Geometry check sheet. Reference: the model listing, model coordinates, mm. A direction names the side the tool comes from. Round coordinates to 2 decimals unless told otherwise and drop trailing zeros. Order: outer loops, then holes, each group sorted by start corner. A loop starts at its lowest first (then second) coordinate and runs counter-clockwise, first axis right, second up. Notation, with made-up numbers: (74, -26.5) - (120, -26.5) arc R33 ccw to (120, 1.5) - close; hole circle Ø3 at (-34.75, -28.5). An arc over 180 degrees is marked (long way). Answer as CSV lines item,"result". Start each with the question number.
```python
from build123d import *

# Parameters (mm, degrees)
SKETCH1_W           = 32
SKETCH1_H           = 22
BOSS_EXTRUDE1_DEPTH = 20
SKETCH2_R           = 4.65
BOSS_EXTRUDE2_DEPTH = 15
SKETCH3_W           = 30
SKETCH3_H           = 20
CUT_EXTRUDE1_DEPTH  = 19
SKETCH4_R           = 2.5
CUT_EXTRUDE2_DEPTH  = 28.166155414
FILLET1_R           = 1
FILLET2_R           = 1
SKETCH5_W           = 30
SKETCH5_H           = 20
SKETCH5_W_2         = 28
SKETCH5_H_2         = 18
BOSS_EXTRUDE3_DEPTH = 14
CUT_EXTRUDE3_REACH  = 50.683
SKETCH8_W           = 8
SKETCH8_H           = 5


with BuildPart() as part:
    # Sketch1 → Boss-Extrude1 (new body)
    with BuildSketch(Plane(origin=(0, 0, 0), x_dir=(1, 0, 0), z_dir=(0, 1, 0))):
        Rectangle(SKETCH1_W, SKETCH1_H)
    extrude(amount=BOSS_EXTRUDE1_DEPTH)

    # Sketch2 → Boss-Extrude2 (add)
    with BuildSketch(Plane(origin=(0, 20, 0), x_dir=(1, 0, 0), z_dir=(0, 1, 0))):
        with Locations(Location((0, 0, 0), (0, 0, 270))):
            Circle(SKETCH2_R)
    extrude(amount=BOSS_EXTRUDE2_DEPTH)

    # Sketch3 → Cut-Extrude1 (cut)
    with BuildSketch(Plane.XZ):
        Rectangle(SKETCH3_W, SKETCH3_H)
    extrude(amount=-CUT_EXTRUDE1_DEPTH, mode=Mode.SUBTRACT)

    # Sketch4 → Cut-Extrude2 (cut, through all)
    with BuildSketch(Plane.XZ.offset(-19)):
        with Locations(Location((0, 0, 0), (0, 0, 270))):
            Circle(SKETCH4_R)
    extrude(amount=-CUT_EXTRUDE2_DEPTH, mode=Mode.SUBTRACT)

    # Fillet1
    fillet1_edges = [part.edges().sort_by_distance(p)[0] for p in [
        (0, 35, -4.65),
    ]]
    fillet(fillet1_edges, radius=FILLET1_R)

    # Fillet2
    fillet2_edges = [part.edges().sort_by_distance(p)[0] for p in [
        (0, 19, 2.5),
    ]]
    fillet(fillet2_edges, radius=FILLET2_R)

    # Sketch5 → Boss-Extrude3 (add)
    with BuildSketch(Plane.XZ.offset(-19)):
        Rectangle(SKETCH5_W, SKETCH5_H)
        Rectangle(SKETCH5_W_2, SKETCH5_H_2, mode=Mode.SUBTRACT)
    extrude(amount=BOSS_EXTRUDE3_DEPTH)

    # Cut-Extrude3: up to this face of the body (flat: up to its plane)
    cut_extrude3_end = Plane(part.part.faces().sort_by_distance((14, 12, 0))[0])
    # Sketch8 → Cut-Extrude3 (cut, up to the picked face)
    with BuildSketch(Plane(origin=(16, 0, 0), x_dir=(0, 0, -1), z_dir=(1, 0, 0)), mode=Mode.PRIVATE) as cut_extrude3_sk1:
        with Locations((0, 5)):
            Rectangle(SKETCH8_W, SKETCH8_H)
    cut_extrude3_tool1 = split(extrude(cut_extrude3_sk1.sketch, amount=-CUT_EXTRUDE3_REACH, mode=Mode.PRIVATE), bisect_by=cut_extrude3_end, keep=Keep.BOTH, mode=Mode.PRIVATE)
    add(cut_extrude3_tool1.solids().sort_by(Axis((16, 5, 0), (-1, 0, 0)))[0], mode=Mode.SUBTRACT)


solid = part.part
```
1. Section check B-B on z = 0. Record the boundary of the cut face in (x, y).
2. Thickness scan on probe 1 along X at (y, z) = (8, -4.75); probe 2 along X at (y, z) = (25.75, 0); probe 3 along Z at (x, y) = (3, 3). Record the ranges inside material, lowest first.
3. Access from +Z, -Z, +X, -X, +Y, -Y to the whole of each face (thin tool, end or side, straight path). Record for faces 5 (the face through (1.397, 26.902, 4.435)), 6 (the face through (0, 2, 10)), 7 (the face through (-2, 35, 2)), 8 (the face through (15, 6, -4)).
4. Draft check along X on faces 1 (the face through (16, 10, 0)), 2 (the face through (0, 2, -10)), 3 (the face through (-1.3, 0, 10.5)), 4 (the face through (14, 12, 0)). Enter one of: released by +X, released by -X, zero draft, split by the parting line, or undercut.
5. Section check D-D on z = -5.5. Record the boundary of the cut face in (x, y).
6. Section check A-A on x = 0. Record the boundary of the cut face in (y, z), plus the area to 3 significant figures.
7. Go/stop test with flat-tipped pins: pin 1 Ø6 at (x, z) = (-1.5, 5) entering from -Y; pin 2 Ø1.5 at (y, z) = (3.5, -2.5) entering from +X; pin 3 Ø0.5 at (x, z) = (15.5, -1.5) entering from +Y. Record where each tip stops, or that it passes through.
8. Section check C-C on y = 11. Record the boundary of the cut face in (x, z), plus the area to 3 significant figures.
Numbers:
1,outline,"(-16, 0) - (-15, 0) - (-15, 5) - (-14, 5) - (-14, 19) - (-3.5, 19) arc R1 ccw to (-2.5, 20) - (-2.5, 35) - (-3.65, 35) arc R1 ccw to (-4.65, 34) - (-4.65, 20) - (-16, 20) - close; (2.5, 20) arc R1 ccw to (3.5, 19) - (14, 19) - (14, 7.5) - (16, 7.5) - (16, 20) - (4.65, 20) - (4.65, 34) arc R1 ccw to (3.65, 35) - (2.5, 35) - close; (15, 0) - (16, 0) - (16, 2.5) - (15, 2.5) - close"
2,probe 1,"x = -16 to -14, 14 to 16"
2,probe 2,"x = -4.65 to -2.5, 2.5 to 4.65"
2,probe 3,"z = -11 to -10, 10 to 11"
3,face 5,"+Y"
3,face 6,"-Y"
3,face 7,"+Z, -Z, +X, -X, +Y"
3,face 8,"+X"
4,face 1,"released by +X"
4,face 2,"undercut"
4,face 3,"zero draft"
4,face 4,"undercut"
5,outline,"(-16, 0) - (-15, 0) - (-15, 5) - (-14, 5) - (-14, 19) - (14, 19) - (14, 5) - (15, 5) - (15, 0) - (16, 0) - (16, 20) - (-16, 20) - close"
6,outline,"(0, -11) - (20, -11) - (20, -4.65) - (34, -4.65) arc R1 ccw to (35, -3.65) - (35, -2.5) - (20, -2.5) arc R1 ccw to (19, -3.5) - (19, -9) - (5, -9) - (5, -10) - (0, -10) - close; (0, 10) - (5, 10) - (5, 9) - (19, 9) - (19, 3.5) arc R1 ccw to (20, 2.5) - (35, 2.5) - (35, 3.65) arc R1 ccw to (34, 4.65) - (20, 4.65) - (20, 11) - (0, 11) - close"
6,area,"147 mm2"
7,pin 1,"stops at y = 19"
7,pin 2,"stops at x = -15"
7,pin 3,"stops at y = 20"
8,outline,"(-16, -11) - (16, -11) - (16, 11) - (-16, 11) - close; hole (-14, -9) - (14, -9) - (14, 9) - (-14, 9) - close"
8,area,"200 mm2"
